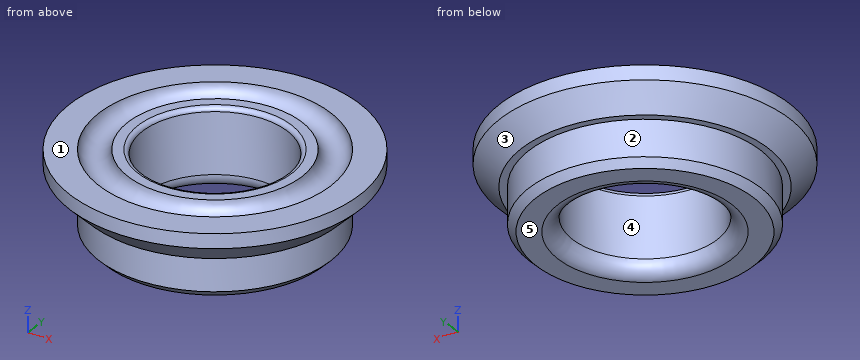
from build123d import *

# Parameters (mm, degrees)
F2_SIZE = 5
F3_R    = 10
F4_R    = 3


with BuildPart() as f1:
    # F0 (on Right) → F1 (revolve)
    with BuildSketch(Plane.YZ):
        with BuildLine():
            Line((60, 0), (50, 0))
            Line((50, 0), (50, -55))
            Line((50, -55), (80, -55))
            Line((80, -55), (80, -25))
            Line((80, -25), (85, -25))
            Line((85, -25), (100, -10))
            Line((100, -10), (100, 0))
            Line((100, 0), (80, 0))
            ThreePointArc((80, 0), (70, -10), (60, 0))
        make_face()
    revolve(axis=Axis((0, 0, -46.653546), (0, 0, -1)))

    # F2
    f2_edges = [f1.edges().sort_by_distance(p)[0] for p in [
        (0, -80, -55),
    ]]
    chamfer(f2_edges, length=F2_SIZE)

    # F3
    f3_edges = [f1.edges().sort_by_distance(p)[0] for p in [
        (0, -50, -55),
    ]]
    fillet(f3_edges, radius=F3_R)

    # F4
    f4_edges = [f1.edges().sort_by_distance(p)[0] for p in [
        (0, -50, 0),
    ]]
    fillet(f4_edges, radius=F4_R)


solid = f1.part
Could you check a few things on this model? Use its own coordinates, in mm. Face numbers are marked on the shaded views. A direction names the side the tool comes from. Give positions to 0.01 mm unless a question says otherwise; leave off trailing zeros. Write each loop counter-clockwise with the first axis right and the second up, starting at its lowest first coordinate (ties: lowest second). Pieces come first, ordered by that corner, then holes. Notation, with made-up numbers: (67.25, 33) -> (116.25, 33) arc R12 ccw to (116.25, 55) -> close; hole circle Ø10 at (-19.75, 83). An arc over 180 degrees is marked (long way). Write each question's results on one line, items separated by ' | '. Start each with the question number.
Q1. I'm going to push flat-ended pins straight in: pin 1 Ø10 at (y, z) = (4.5, -15.5) entering from -X; pin 2 Ø4 at (x, z) = (46, -11.5) entering from +Y; pin 3 Ø1 at (y, z) = (8, -12.5) entering from -X. Where does each tip first touch, or does it pass through?
Q2. I need wall thicknesses on probe 1 along X at (y, z) = (0, -27); probe 2 along Y at (x, z) = (54.5, -7.5); probe 3 along X at (y, z) = (21, -8). Which ranges of each line are inside material? Lowest first, please.
Q3. We'd pull the mould along Y, two halves only. Please class the marked faces 3, 4 and 5: +Y half, -Y half, draft (parallel to the pull), parting line (faces both ways), or undercut.
Q4. Suppose I cut it at C-C, the plane z = -22. List the corners of the cut face in (x, y) for me, and give its area (3 significant figures).
Q5. Suppose I cut it at A-A, the plane y = 0. List the corners of the cut face in (x, z) for me, and give its area (3 significant figures).
Q6. Which directions (+Z, -Z, +X, -X, +Y, -Y) give clear straight access to the entire face, cutting with the end or side of a thin tool? Please do the marked faces 1 and 2.
Outcome:
1) pin 1: x = -99.4 | pin 2: y = 89.46 | pin 3: x = -97.67
2) probe 1: -80 to -50, 50 to 80 | probe 2: -83.84 to -53.85, -32.36 to 32.36, 53.85 to 83.84 | probe 3: -97.77 to -73.04, -60.46 to -45.38, 45.38 to 60.46, 73.04 to 97.77
3) face 3: parting line | face 4: undercut | face 5: draft
4) outline: circle Ø176 at (0, 0); hole circle Ø100 at (0, 0) | area: 16,500 mm2
5) outline: (-100, -10) -> (-85, -25) -> (-80, -25) -> (-80, -50) -> (-75, -55) -> (-60, -55) arc R10 ccw to (-50, -45) -> (-50, -3) arc R3 ccw to (-53, 0) -> (-60, 0) arc R10 cw to (-80, 0) -> (-100, 0) -> close; (50, -45) arc R10 ccw to (60, -55) -> (75, -55) -> (80, -50) -> (80, -25) -> (85, -25) -> (100, -10) -> (100, 0) -> (80, 0) arc R10 cw to (60, 0) -> (53, 0) arc R3 ccw to (50, -3) -> close | area: 3,690 mm2
6) face 1: +Z, +X, -X, +Y, -Y | face 2: -Z
